The listing builds one solid part. Answer for the finished solid, in the listing's coordinates (mm). Face numbers are marked on the shaded views. A direction names the side the tool comes from. Give positions to 0.01 mm unless a question says otherwise; leave off trailing zeros. Write each loop counter-clockwise with the first axis right and the second up, starting at its lowest first coordinate (ties: lowest second). Pieces come first, ordered by that corner, then holes. Notation, with made-up numbers: (60.25, -13) - (99.25, -13) arc R23 cw to (99.25, 16) - close; hole circle Ø6 at (29.5, 47). An arc over 180 degrees is marked (long way). Return JSON: item names as keys, results as strings.
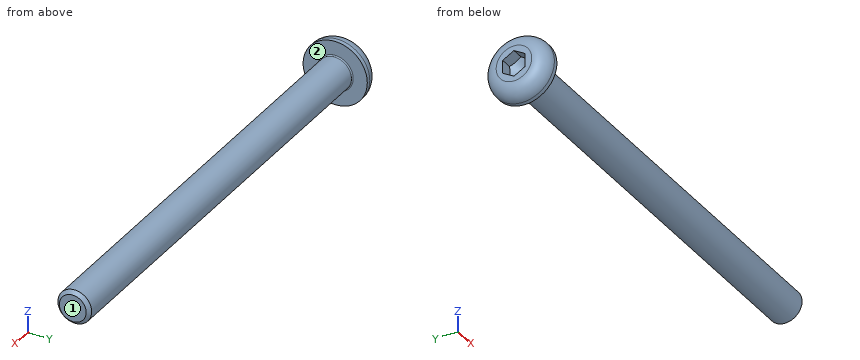
Autodesk Inventor part; units mm, degrees
ref_plane "Work Plane1" through (30, 0, 0) normal (0, -0.5, 0.866) x (1, 0, 0)
ref_plane "YZ Plane" through (0, 0, 0) normal (1, 0, 0) x (0, 1, 0)
ref_plane "XZ Plane" through (0, 0, 0) normal (0, 1, 0) x (-1, 0, 0)
sketch "Sketch1" plane through (0, 0, 0) normal (0, 0, 1) x (1, 0, 0)
  line L0 (0.0567, 0) -> (40, 0)
  line L1 (40, 0) -> (40, 1.5)
  line L2 (40, 1.5) -> (1, 1.5)
  line L3 (1, 1.5) -> (0.6933, 1.5)
  line L4 (0.6933, 1.5) -> (0, 1.5)
  line L5 (0, 1.5) -> (0, 2.85)
  line L6 (0, 2.85) -> (-1.65, 2.85)
  line L7 (-1.65, 2.85) -> (-1.65, 1.1547)
  line L8 (-1.65, 1.1547) -> (-0.61, 1.1547)
  line L9 (-0.61, 1.1547) -> (0.0567, 0)
  line L10 (-9.98, 0) -> (48.33, 0)
  line L11 (0, -0.57) -> (0, 3.42)
  line L12 (1, 1.5) -> (0, 1.5) construction
  dimension "d0" = 39
  dimension "d1" = 0.3067
  dimension "d2" = 1.65
  dimension "d3" = 1.04
  dimension "d4" = 60
  dimension "d5" = 3
  dimension "d6" = 3
  dimension "d7" = 2.3094
  dimension "d8" = 5.7
  dimension "d19" = 40
revolve "Body" add sketch "Sketch1" angle 360 about axis through (0.0567, 0, 0) along (1, 0, 0) contours L9 L11 L4 L3 L2 L1 L0 | L9 L8 L7 L6 L5 L11
sketch "Sketch2" plane through (-1.65, 0, 0) normal (-1, 0, 0) x (0, 0, 1)
  circle A0 centre (0, 0) radius 1.1547
  line L0 (0, -3.99) -> (0, 3.99)
  line L1 (-3.99, 0) -> (3.99, 0)
  line L2 (1.1547, 0) -> (0.5774, -1)
  line L3 (0.5774, -1) -> (-0.5774, -1)
  line L4 (-0.5774, -1) -> (-1.1547, 0)
  line L5 (-1.1547, 0) -> (-0.5774, 1)
  line L6 (-0.5774, 1) -> (0.5774, 1)
  line L7 (0.5774, 1) -> (1.1547, 0)
extrude "Slot" add sketch "Sketch2" against normal up to next contours L7 A0 | A0 L2 | L6 L0 A0 | A0 L0 L3 | L0 L6 A0 | A0 L3 L0 | L4 A0 | A0 L5
fillet "Fillet1" radius 1.27 1 edges at (-1.65, -2.85, 0)
thread "Thread"
chamfer "Chamfer1" distance 0.3067 distance2 0.3067 1 edges at (40, -1.5, 0) measured on face at (40, -0.1088, 0.5667)
fillet "Fillet2" radius 0.1 1 edges at (0, -1.5, 0)
ref_plane "Work Plane1" through (30, 0, 0) normal (0, -0.5, 0.866) x (1, 0, 0)
equation "\"d16\" = RR"
equation "\"d12\" = GEL"
equation "\"d14\" = -0.5 * SPD + 0.5 * GD"
equation "\"d15\" = GUL"
equation "\"d29\" = R"
equation "\"d0\" = GEL"
equation "\"d1\" = GAL"
equation "\"d2\" = KOH"
equation "\"d3\" = INTI"
equation "\"d5\" = GD"
equation "\"d6\" = BDM"
equation "\"d7\" = 1.1547 * SW"
equation "\"d8\" = KOD"
equation "\"d19\" = NLG"
equation "\"GD\" = NND"
equation "\"NLG\" = 40"
equation "\"GEL\" = 39"
equation "\"KOD\" = 5.7"
equation "\"KOH\" = 1.65"
equation "\"INTI\" = 1.04"
equation "\"GAL\" = 0.61345 * PTC"
equation "\"GUL\" = 0.61345 * PTC"
equation "\"BDM\" = NND"
equation "\"SW\" = 2"
equation "\"RR\" = 1.27"
equation "\"SPD\" = 2.38655"
equation "\"d28\" = R"
equation "\"R\" = 0.1"
equation "\"TOA\" = 30deg"
equation "\"THREADDIA\" = 3"
equation "\"KOD1\" = KOD - 2 * RR"
equation "\"PTC\" = 0.5"
equation "\"NND\" = 3"
equation "\"E0\" = 1.155 * SW"
equation "\"GD1\" = THREADDIA - 1.2269 * PTC"
properties part number "ANSI B18.3.4M - M3 x 0.5 x 40, FHSBHCSM" material "Steel, Mild"
Item 1: For the marked faces 1 and 2, determine the directions among +Z, -Z, +X, -X, +Y, -Y from which every point of the face is accessible in a straight line to the end or side of a thin tool.
Answer below:
{"face 1": "+Z, -Z, +X, +Y, -Y", "face 2": "+X"}
Item 2: A cutting plane is placed at A-A on x = 6. Determine the outline of the cut face in (y, z).
Answer below:
{"outline": "circle Ø3 at (0, 0)"}
Item 3: Flat-ended cylindrical pins translate along their axes: P1, Ø1.5, axis at x = 19.5, y = 2, coming from the +Z side; P2, Ø2, axis at y = -2, z = -2, coming from the +X side; P3, Ø2, axis at x = 11, y = 2, coming from the -Z side. Find the tip coordinate at first contact, or state that the pin passes through.
Answer below:
{"P1": "stops at z = 0.83", "P2": "stops at x = 0", "P3": "stops at z = -1.12"}
Item 4: Consider L1, parallel to Y at x = 15.5, z = 0.15; L2, parallel to X at y = 1, z = 2.5; L3, parallel to Z at x = 24, y = -0.95. Determine where each line is inside the solid, lowest interval first.
Answer below:
{"L1": "y = -1.49 to 1.49", "L2": "x = -0.99 to 0", "L3": "z = -1.16 to 1.16"}
